Verification items for the finished model (mm, model axes). A direction names the side the tool comes from. Coordinates: 2 decimals unless noted, no trailing zeros. Loops run counter-clockwise (first coordinate to the right, second up) from the corner with the lowest first, then second, coordinate; pieces in that order, holes last. Notation, with made-up numbers: (18.25, 68) -> (32.25, 68) arc R29 cw to (32.25, 88) -> close; hole circle Ø3 at (-17, -17.5). An arc over 180 degrees is marked (long way). Write item = value, one per line.
```python
from build123d import *

# Parameters (mm, degrees)
F0_W     = 50.8
F0_H     = 50.8
F1_DEPTH = 12.7
F2_R     = 12.7
F3_DEPTH = 76.2
F4_SIZE  = 2.54
F5_W     = 25.4
F5_H     = 50.8
F6_DEPTH = 76.2
F7_R     = 9.525
F8_DEPTH = 38.101


with BuildPart() as f1:
    # F0 (on Right) → F1 (new body)
    with BuildSketch(Plane.YZ):
        with Locations((25.4, 25.4)):
            Rectangle(F0_W, F0_H)
    extrude(amount=F1_DEPTH)

    # F2 (on face) → F3 (join)
    with BuildSketch(Plane.YZ.offset(12.7)):
        with Locations((25.4, 25.4)):
            Circle(F2_R)
    extrude(amount=F3_DEPTH)

    # F4
    f4_edges = [f1.edges().sort_by_distance(p)[0] for p in [
        (88.9, 12.7, 25.4),
    ]]
    chamfer(f4_edges, length=F4_SIZE)

    # F5 (on face) → F6 (join)
    with BuildSketch(Plane(origin=(0, 0, 0), x_dir=(0, -1, 0), z_dir=(-1, 0, 0))):
        with Locations((-25.4, 25.4)):
            Rectangle(F5_W, F5_H)
    extrude(amount=F6_DEPTH)

    # F7 (on face) → F8 (cut, through all)
    with BuildSketch(Plane.XZ.offset(-12.7)):
        with BuildLine():
            ThreePointArc((-76.2, 25.4), (-68.760512, 43.360512), (-50.8, 50.8))
            Line((-50.8, 50.8), (-76.2, 50.8))
            Line((-76.2, 50.8), (-76.2, 25.4))
        make_face()
        with BuildLine():
            ThreePointArc((-50.8, 0), (-68.760512, 7.439488), (-76.2, 25.4))
            Line((-76.2, 25.4), (-76.2, 0))
            Line((-76.2, 0), (-50.8, 0))
        make_face()
        with Locations((-50.8, 25.4)):
            Circle(F7_R)
    extrude(amount=-F8_DEPTH, mode=Mode.SUBTRACT)


solid = f1.part
```
1) Release check for a two-part mould opening along Z. For faces 1 (the face through (49.014, 16.04, 33.983)), 2 (the face through (-38, 12.7, 25)), 3 (the face through (-46.4, 25.22, 16.95)) record: pulls with the +Z half, pulls with the -Z half, needs draft (parallel to the pull), parting line crosses it, or undercut.
Ans:
face_1 = parting line crosses it
face_2 = needs draft
face_3 = undercut
2) Depth check by flat-ended pin: pin 1 Ø22 at (x, z) = (-50.8, 25.4) entering from -Y; pin 2 Ø10 at (y, z) = (14, 35.5) entering from -X; pin 3 Ø1 at (x, y) = (64.5, 17.5) entering from +Z. Enter the tip coordinate at first touch or a pass-through.
Ans:
pin_1 = 12.7
pin_2 = -75.68
pin_3 = 35.72
3) Tool access check on faces 4 (the face through (-12, 25, 50.8)), 5 (the face through (0, 6, 26)), 6 (the face through (6, 0, 25)), 7 (the face through (-38, 38.1, 25)), 8 (the face through (12.7, 19, 37)). Record the directions out of +Z, -Z, +X, -X, +Y, -Y that give a thin tool (end or side, any length) a straight path to the whole face; none if there is none.
Ans:
face_4 = +Z, +X, -X, +Y, -Y
face_5 = +Z, -Z, -X, -Y
face_6 = +Z, -Z, +X, -X, -Y
face_7 = +Z, -Z, -X, +Y
face_8 = +X
4) Sectioned sample at A-A, the plane y = 25.4. Record the cut outline in (x, z) (3 decimals).
Ans:
outline = (-76.2, 25.4) arc R25.4 ccw to (-50.8, 0) -> (12.7, 0) -> (12.7, 12.7) -> (86.36, 12.7) -> (88.9, 15.24) -> (88.9, 35.56) -> (86.36, 38.1) -> (12.7, 38.1) -> (12.7, 50.8) -> (-50.8, 50.8) arc R25.4 ccw to start; hole circle Ø19.05 at (-50.8, 25.4)
5) Material ranges on line 1 (Z direction, x = -50, y = 19); line 2 (X direction, y = 32, z = 25); line 3 (Y direction, x = -24, z = 11.5), recorded low to high.
Ans:
line_1 = 0 to 15.91, 34.89 to 50.8
line_2 = -76.2 to -60.32, -41.28 to 88.9
line_3 = 12.7 to 38.1
6) Sectioned sample at B-B, the plane x = -29. Record the cut outline in (y, z), plus the area to 3 significant figures.
Ans:
outline = (12.7, 0) -> (38.1, 0) -> (38.1, 50.8) -> (12.7, 50.8) -> close
area = 1,290 mm2
